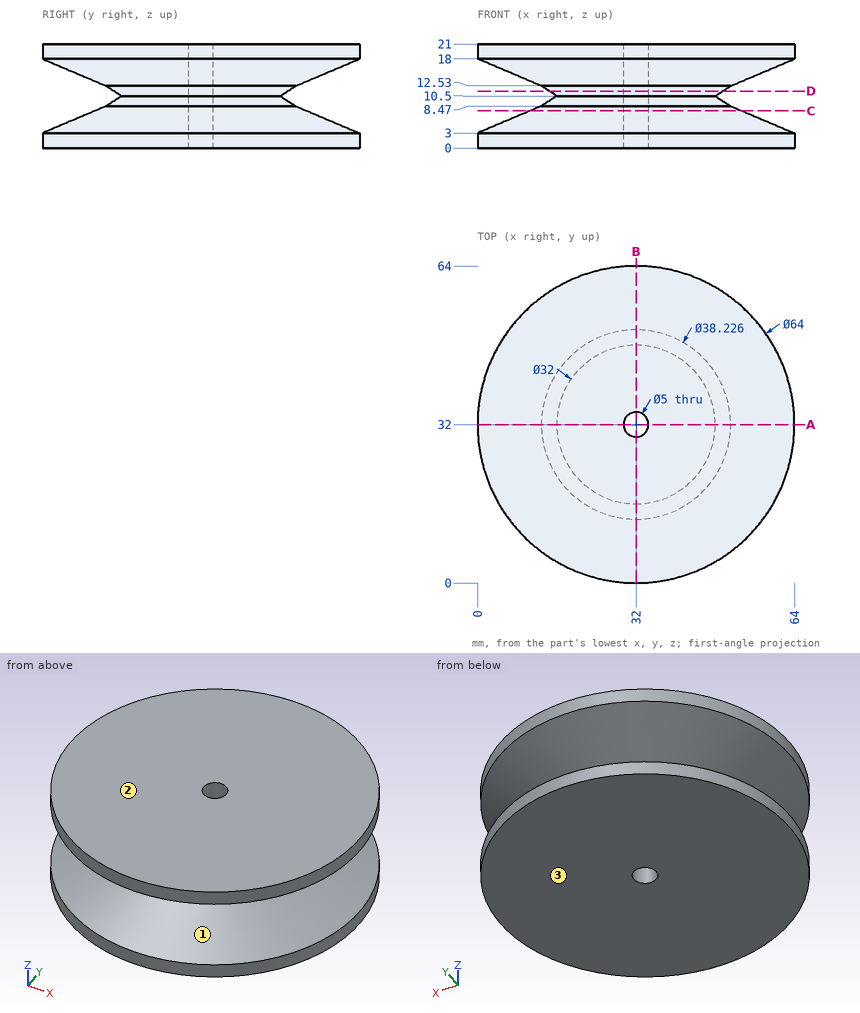
Geometry check sheet. Reference: drawing and pictorial views, mm from the part's lowest x, y, z. Give positions to 0.01 mm unless a question says otherwise; leave off trailing zeros. Write each loop counter-clockwise with the first axis right and the second up, starting at its lowest first coordinate (ties: lowest second). Pieces come first, ordered by that corner, then holes. Notation, with made-up numbers: (0.25, -5.75) -> (26.25, -5.75) arc R8 cw to (26.25, 6.25) -> close; hole circle Ø3 at (-14.5, 79.5). An arc over 180 degrees is marked (long way). One line per question, with ' | ' between items.
Item 1: Sectioned sample at D-D, the plane z = 11.5. Record the boundary of the cut face in (x, y), plus the area to 3 significant figures.
Determined:
outline: circle Ø35.07 at (32, 32); hole circle Ø5 at (32, 32) | area: 946 mm^2
Item 2: Draft check along Z on the marked faces 1, 2 and 3. Enter one of: released by +Z, released by -Z, zero draft, split by the parting line, or undercut.
Determined:
face 1: undercut | face 2: released by +Z | face 3: released by -Z
Item 3: Scan lines: line 1 along X through (y, z) = (32, 14) (1 decimal); line 2 along Z through (x, y) = (50, 48); line 3 along Y through (x, z) = (32, 16.75) (1 decimal). Record each from-to range of solid material in increasing order.
Determined:
line 1: 9.4 to 29.5, 34.5 to 54.6 | line 2: 0 to 6.36, 14.64 to 21 | line 3: 2.9 to 29.5, 34.5 to 61.1
Item 4: Sectioned sample at A-A, the plane y = 32. Record the boundary of the cut face in (x, z).
Determined:
outline: (0, 0) -> (29.5, 0) -> (29.5, 21) -> (0, 21) -> (0, 18) -> (12.89, 12.53) -> (16, 10.5) -> (12.89, 8.47) -> (0, 3) -> close; (34.5, 0) -> (64, 0) -> (64, 3) -> (51.11, 8.47) -> (48, 10.5) -> (51.11, 12.53) -> (64, 18) -> (64, 21) -> (34.5, 21) -> close
Item 5: Depth check by flat-ended pin: pin 1 (12 mm diameter, centred on y = 34.5, z = 12.5, fed in from +X); pin 2 (6 mm diameter, centred on y = 39, z = 10, fed in from +X) (1 decimal); pin 3 (3 mm diameter, centred on x = 30.5, z = 5.5, fed in from +Y). Enter the tip coordinate at first touch or a pass-through.
Determined:
pin 1: x = 64 | pin 2: x = 53.5 | pin 3: y = 61.61
Item 6: Sectioned sample at C-C, the plane z = 7.5. Record the boundary of the cut face in (x, y).
Determined:
outline: circle Ø42.8 at (32, 32); hole circle Ø5 at (32, 32)
